```python
from build123d import *

# Parameters (mm, degrees)
F0_W     = 36
F0_H     = 25
F1_DEPTH = 35
F2_W     = 20.5
F2_H     = 25
F3_DEPTH = 25
F4_R     = 1
F5_R     = 5
F6_W     = 8
F6_H     = 6
F7_DEPTH = 3
F8_W     = 8
F8_H     = 6
F9_DEPTH = 3


with BuildPart() as f1:
    # F0 (on Top) → F1 (new body)
    with BuildSketch(Plane.XY):
        with Locations((18, 12.5)):
            Rectangle(F0_W, F0_H)
    extrude(amount=F1_DEPTH)

    # F2 (on face) → F3 (cut)
    with BuildSketch(Plane.XY.offset(35)):
        with Locations((18, 12.5)):
            Rectangle(F2_W, F2_H)
    extrude(amount=-F3_DEPTH, mode=Mode.SUBTRACT)

    # F4
    f4_edges = [f1.edges().sort_by_distance(p)[0] for p in [
        (0, 0, 17.5),
        (0, 12.5, 35),
        (0, 25, 17.5),
        (36, 25, 17.5),
        (36, 12.5, 35),
        (36, 0, 17.5),
    ]]
    fillet(f4_edges, radius=F4_R)

    # F5
    f5_edges = [f1.edges().sort_by_distance(p)[0] for p in [
        (7.75, 12.5, 10),
        (28.25, 12.5, 10),
    ]]
    fillet(f5_edges, radius=F5_R)

    # F6 (on face) → F7 (cut)
    with BuildSketch(Plane(origin=(0, 0, 0), x_dir=(0, -1, 0), z_dir=(-1, 0, 0))):
        with Locations((-12.5, 29)):
            Rectangle(F6_W, F6_H)
    extrude(amount=-F7_DEPTH, mode=Mode.SUBTRACT)

    # F8 (on face) → F9 (cut)
    with BuildSketch(Plane.YZ.offset(36)):
        with Locations((12.5, 29)):
            Rectangle(F8_W, F8_H)
    extrude(amount=-F9_DEPTH, mode=Mode.SUBTRACT)


solid = f1.part
```
Geometry: final body of the model. Coordinates: model frame, mm. A direction names the side the tool comes from. Round coordinates to 2 decimals unless told otherwise and drop trailing zeros. Write each loop counter-clockwise with the first axis right and the second up, starting at its lowest first coordinate (ties: lowest second). Pieces come first, ordered by that corner, then holes. Notation, with made-up numbers: (8.5, 69) -> (48.5, 69) arc R25 cw to (48.5, 99) -> close; hole circle Ø10 at (75.5, 3). An arc over 180 degrees is marked (long way). Return JSON: item names as keys, results as strings.
Q1. Set-up query: faces 1 (the cylindrical face through (35.699, 24.715, 17.745)), 2 (the flat face through (35, 12, 32)), 3 (the flat face through (1, 8.5, 29)). Return all of +Z, -Z, +X, -X, +Y, -Y with unobstructed straight access to the full face (end or side cutting, diameter ignored); none if empty.
From the geometry:
{"face 1": "+Z, -Z, +X, +Y", "face 2": "+X", "face 3": "-X"}
Q2. Section C-C on y = 10.75. Return the cut outline in (x, z).
From the geometry:
{"outline": "(0, 0) -> (36, 0) -> (36, 26) -> (33, 26) -> (33, 32) -> (36, 32) -> (36, 34) arc R1 ccw to (35, 35) -> (28.25, 35) -> (28.25, 15) arc R5 cw to (23.25, 10) -> (12.75, 10) arc R5 cw to (7.75, 15) -> (7.75, 35) -> (1, 35) arc R1 ccw to (0, 34) -> (0, 32) -> (3, 32) -> (3, 26) -> (0, 26) -> close"}
Q3. Ray query, line 1 (X direction, y = 22.25, z = 24); line 2 (Z direction, x = 21, y = 7.5); line 3 (X direction, y = 23, z = 10.5). Return the intervals inside material, ascending.
From the geometry:
{"line 1": "0 to 7.75, 28.25 to 36", "line 2": "0 to 10", "line 3": "0 to 10.57, 25.43 to 36"}
Q4. First-contact query: pin 1 Ø10 at (x, y) = (21.5, 18) entering from +Z; pin 2 Ø1.8 at (y, z) = (14, 29.5) entering from +X; pin 3 Ø8.5 at (x, y) = (16, 14.5) entering from +Z. Flat tips, straight axial feed; report the tip coordinate or a pass-through.
From the geometry:
{"pin 1": "z = 11.2", "pin 2": "x = 33", "pin 3": "z = 10.1"}
Q5. Section A-A on z = 31.5. Return the cut outline in (x, y).
From the geometry:
{"outline": "(0, 1) arc R1 ccw to (1, 0) -> (7.75, 0) -> (7.75, 25) -> (1, 25) arc R1 ccw to (0, 24) -> (0, 16.5) -> (3, 16.5) -> (3, 8.5) -> (0, 8.5) -> close; (28.25, 0) -> (35, 0) arc R1 ccw to (36, 1) -> (36, 8.5) -> (33, 8.5) -> (33, 16.5) -> (36, 16.5) -> (36, 24) arc R1 ccw to (35, 25) -> (28.25, 25) -> close"}
Q6. Section B-B on z = 18. Return the cut outline in (x, y).
From the geometry:
{"outline": "(0, 1) arc R1 ccw to (1, 0) -> (7.75, 0) -> (7.75, 25) -> (1, 25) arc R1 ccw to (0, 24) -> close; (28.25, 0) -> (35, 0) arc R1 ccw to (36, 1) -> (36, 24) arc R1 ccw to (35, 25) -> (28.25, 25) -> close"}
Q7. Section D-D on y = 5.25. Return the cut outline in (x, z), and give its area (3 significant figures).
From the geometry:
{"outline": "(0, 0) -> (36, 0) -> (36, 34) arc R1 ccw to (35, 35) -> (28.25, 35) -> (28.25, 15) arc R5 cw to (23.25, 10) -> (12.75, 10) arc R5 cw to (7.75, 15) -> (7.75, 35) -> (1, 35) arc R1 ccw to (0, 34) -> close", "area": "758 mm2"}
Q8. Mould query, pull axis Z, two halves, no side actions, for faces 4 (the flat face through (1, 13, 32)), 5 (the flat face through (7.75, 12, 25)), 6 (the cylindrical face through (9.18, 12.68, 11.5)), 7 (the flat face through (1, 16.5, 29)). Classes: +Z half, -Z half, draft (parallel to the pull), parting line (faces both ways), or undercut.
From the geometry:
{"face 4": "undercut", "face 5": "draft", "face 6": "+Z half", "face 7": "undercut"}
